Verification items for this drawing (mm, ordinates from the low corner). Give positions to 0.01 mm unless a question says otherwise; leave off trailing zeros. Order: outer loops, then holes, each group sorted by start corner. A loop starts at its lowest first (then second) coordinate and runs counter-clockwise, first axis right, second up. Notation, with made-up numbers: (34, 35.25) -> (92, 35.25) arc R9 ccw to (92, 45.25) -> close; hole circle Ø9 at (28.25, -29.5). An arc over 180 degrees is marked (long way). One line per question, with ' | ' between items.
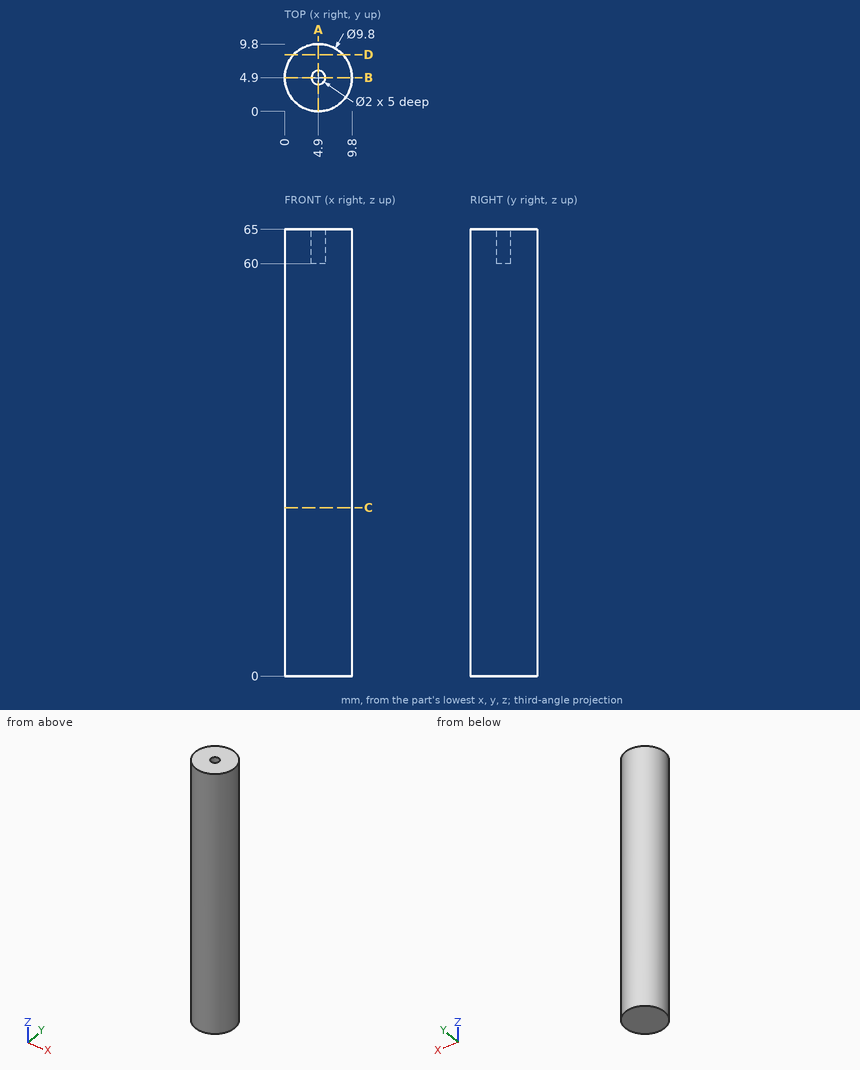
Q1. Section check D-D (y = 8.25). Enter the section's corners in (x, z), and give its area (3 significant figures).
Result sheet:
outline: (1.32, 0) -> (8.48, 0) -> (8.48, 65) -> (1.32, 65) -> close | area: 465 mm2
Q2. Section check C-C (z = 24.5). Enter the section's corners in (x, y).
Result sheet:
outline: circle Ø9.8 at (4.9, 4.9)
Q3. Depth check by flat-ended pin: pin 1 Ø1 at (x, y) = (5.5, 5) entering from +Z; pin 2 Ø3 at (y, z) = (2.5, 25.5) entering from -X; pin 3 Ø3 at (x, z) = (2.5, 48.5) entering from +Y; pin 4 Ø1 at (x, z) = (7.5, 29.5) entering from +Y. Enter the tip coordinate at first touch or a pass-through.
Result sheet:
pin 1: stops at z = 65 | pin 2: stops at x = 0.08 | pin 3: stops at y = 9.72 | pin 4: stops at y = 9.33
Q4. Section check A-A (x = 4.9). Enter the section's corners in (y, z).
Result sheet:
outline: (0, 0) -> (9.8, 0) -> (9.8, 65) -> (5.9, 65) -> (5.9, 60) -> (3.9, 60) -> (3.9, 65) -> (0, 65) -> close
Q5. Thickness scan on line 1 (Y direction, x = 4.9, z = 62.6); line 2 (X direction, y = 5, z = 13); line 3 (Y direction, x = 0.75, z = 11). Record the ranges inside material, lowest first.
Result sheet:
line 1: y = 0 to 3.9, 5.9 to 9.8 | line 2: x = 0 to 9.8 | line 3: y = 2.29 to 7.51
